Input: part model. Units: mm. Frame: model coordinates. Coordinates: 2 decimals unless noted, no trailing zeros. Write each loop counter-clockwise with the first axis right and the second up, starting at its lowest first coordinate (ties: lowest second). Pieces come first, ordered by that corner, then holes.
1) Section query A-A (z = -4.75). Output: boundary loops of the cut face in (x, y).
2) Section query B-B (x = 27). Output: boundary loops of the cut face in (y, z), then the cut area to 3 significant figures.
3) Line query: L1, parallel to X at y = -0.5, z = -4.25; L2, parallel to X at y = 0.8, z = 5.25; L3, parallel to Z at x = -80.85, y = 0. Output: solid intervals per line, ascending.
4) Pin query (flat end, axial travel): pin 1 Ø1.5 at (y, z) = (0.5, 6) entering from -X; pin 2 Ø2.5 at (x, y) = (41, -1) entering from +Z; pin 3 Ø1.5 at (y, z) = (0, -6.5) entering from +X. Return the tip coordinate at first contact, or that it passes through.
from build123d import *

# Parameters (mm, degrees)
SKETCH_W      = 170
SKETCH_H      = 5
PAD_DEPTH     = 2
SKETCH001_W   = 3
SKETCH001_H   = 5
PAD001_DEPTH  = 5.5
FILLET_R      = 2.49
SKETCH002_R   = 0.75
POCKET_DEPTH  = 200
SKETCH003_W   = 3
SKETCH003_H   = 5
SKETCH003_W_2 = 6
PAD002_DEPTH  = 10


with BuildPart() as part:
    # Sketch → Pad (new body)
    with BuildSketch(Plane.XY):
        Rectangle(SKETCH_W, SKETCH_H)
    extrude(amount=PAD_DEPTH)

    # Sketch001 (on Face6 of Pad) → Pad001 (join)
    with BuildSketch(Plane.XY.offset(2)):
        with Locations((-80.3, 0)):
            Rectangle(SKETCH001_W, SKETCH001_H)
        with Locations((80.3, 0)):
            Rectangle(SKETCH001_W, SKETCH001_H)
        with Locations((-4.7, 0)):
            Rectangle(SKETCH001_W, SKETCH001_H)
        with Locations((4.7, 0)):
            Rectangle(SKETCH001_W, SKETCH001_H)
    extrude(amount=PAD001_DEPTH)

    # Fillet
    fillet_edges = [part.edges().sort_by_distance(p)[0] for p in [
        (-80.3, -2.5, 7.5),
        (-4.7, -2.5, 7.5),
        (4.7, -2.5, 7.5),
        (80.3, -2.5, 7.5),
        (80.3, 2.5, 7.5),
        (4.7, 2.5, 7.5),
        (-4.7, 2.5, 7.5),
        (-80.3, 2.5, 7.5),
    ]]
    fillet(fillet_edges, radius=FILLET_R)

    # Sketch002 (on Face29 of Fillet) → Pocket (cut)
    with BuildSketch(Plane.YZ.offset(81.8)):
        with Locations((0, 5)):
            Circle(SKETCH002_R)
    extrude(amount=-POCKET_DEPTH, mode=Mode.SUBTRACT)

    # Sketch003 (on Face13 of Pocket) → Pad002 (join)
    with BuildSketch(Plane(origin=(0, 0, 0), x_dir=(1, 0, 0), z_dir=(0, 0, -1))):
        with Locations((-80.4, 0)):
            Rectangle(SKETCH003_W, SKETCH003_H)
        Rectangle(SKETCH003_W_2, SKETCH003_H)
        with Locations((80.4, 0)):
            Rectangle(SKETCH003_W, SKETCH003_H)
    extrude(amount=PAD002_DEPTH)


solid = part.part
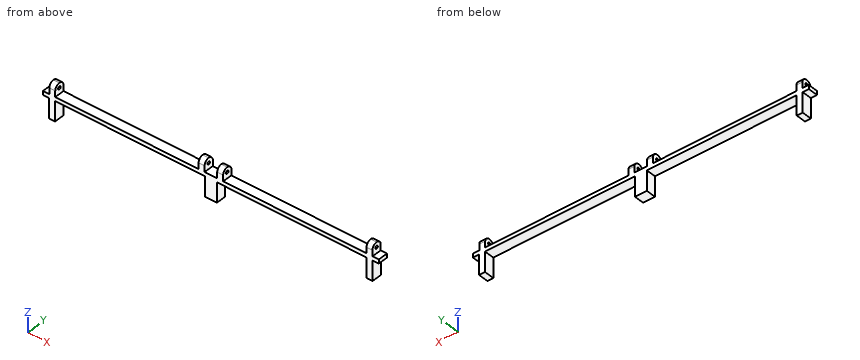
Answer:
1. outline: (-81.9, -2.5) - (-78.9, -2.5) - (-78.9, 2.5) - (-81.9, 2.5) - close; (-3, -2.5) - (3, -2.5) - (3, 2.5) - (-3, 2.5) - close; (78.9, -2.5) - (81.9, -2.5) - (81.9, 2.5) - (78.9, 2.5) - close
2. outline: (-2.5, 0) - (2.5, 0) - (2.5, 2) - (-2.5, 2) - close
2. area: 10.0 mm2
3. L1: x = -81.9 to -78.9, -3 to 3, 78.9 to 81.9
3. L2: x = -81.8 to -78.8, -6.2 to -3.2, 3.2 to 6.2, 78.8 to 81.8
3. L3: z = -10 to 4.25, 5.75 to 7.5
4. pin 1: stops at x = -81.8
4. pin 2: stops at z = 2
4. pin 3: stops at x = 81.9
